Can you work these out from the model? Positions are in its coordinate system, mm. A direction names the side the tool comes from. Coordinates: 2 decimals unless noted, no trailing zeros. Order: outer loops, then holes, each group sorted by start corner. A loop starts at its lowest first (then second) coordinate and runs counter-clockwise, first axis right, second up. Notation, with made-up numbers: (49.5, 78) -> (84.5, 78) arc R35 ccw to (84.5, 114) -> close; hole circle Ø6 at (-18, 25). An arc over 180 degrees is marked (long way). Return JSON: item names as keys, results as strings. Group by question number.
1) If I drill on probe 1 along Y at (x, z) = (-17.5, 2.45); probe 2 along Y at (x, z) = (-12, 2.5); probe 3 along X at (y, z) = (27, 1.75), over which ranges is the centre line in solid material (lowest first)? Write a range as from..to.
2) If we section it at C-C, the plane z = 1.9: State how many separate pieces and enclosed holes the cut face has, then the cut area to 3 significant figures.
3) For pin 1 (1.5 mm diameter, centred on y = 46.5, z = 1.5, fed in from +X); pin 2 (1 mm diameter, centred on x = -18.5, z = 2, fed in from -Y); pin 3 (1 mm diameter, centred on y = -7.5, z = 1.5, fed in from -X), each with a flat end and sliding along its axis, tell me the tip position at first contact or that it passes through.
4) If we section it at A-A, the plane y = 19.2: Please give me the cut outline in (x, z) (3 decimals).
5) Thinking about a two-plate mould opening in X: for faces 3 (the cylindrical face through (-0.6, -8.93, 1.61)), 4 (the cylindrical face through (-19.66, 56.19, 2.1)), 5 (the cylindrical face through (-9.11, 6.47, 1.61)), which applies, +X half, -X half, draft (parallel to the pull), parting line (faces both ways), or undercut?
6) If we section it at D-D, the plane y = 4: Please give me the cut outline in (x, z) (3 decimals), then the cut area to 3 significant figures.
7) If we section it at B-B, the plane x = -12: Please give me the cut outline in (y, z) (3 decimals), then the cut area to 3 significant figures.
8) For faces 1 (the cylindrical face through (-19.41, 31.24, 2.1)), 2 (the flat face through (-20, 9.89, 2)), which set-ups out of +Z, -Z, +X, -X, +Y, -Y let a thin tool reach every point of the face, with its end or its side?
from build123d import *

# Parameters (mm, degrees)
SKETCH1_R                                       = 2.5
SKETCH1_R_2                                     = 5
SKETCH1_R_3                                     = 1
BOSS_EXTRUDE1_DEPTH                             = 3.175
CSK_FOR_M2_FLAT_HEAD_MACHINE_SCREW1_D           = 2.4
CSK_FOR_M2_FLAT_HEAD_MACHINE_SCREW1_CSINK_D     = 4.4
CSK_FOR_M2_FLAT_HEAD_MACHINE_SCREW1_CSINK_ANGLE = 90
SKETCH6_W                                       = 8
SKETCH6_H                                       = 3.2
MOTORSHAFTCUTOUT_DEPTH                          = 68.698453638
F_5MM_FILLET_R                                  = 5
F_1MM_FILLET_R                                  = 1
CUT_EXTRUDE1_DEPTH                              = 68.698453638
FILLET1_R                                       = 5
SKETCH8_W                                       = 5.5
SKETCH8_H                                       = 4
BOSS_EXTRUDE2_DEPTH                             = 3.175
BOSS_EXTRUDE3_DEPTH                             = 3.175
CUT_EXTRUDE3_DEPTH                              = 68.698453638
CUT_EXTRUDE3_DEPTH_BACK                         = 10
FILLET3_R                                       = 12
FILLET4_R                                       = 2
FILLET6_R                                       = 13
CSK_FOR_M2_FLAT_HEAD_MACHINE_SCREW3_D           = 2.4
CSK_FOR_M2_FLAT_HEAD_MACHINE_SCREW3_CSINK_D     = 4.4
CSK_FOR_M2_FLAT_HEAD_MACHINE_SCREW3_CSINK_ANGLE = 90


with BuildPart() as part:
    # Sketch1 → Boss-Extrude1 (new body)
    with BuildSketch(Plane.XY):
        with BuildLine():
            Line((0, -5.5), (-7, -5.5))
            Line((-7, -5.5), (-7, -9))
            Line((-7, -9), (-12, -9))
            Line((-12, -9), (-12, -2.5))
            Line((-12, -2.5), (-27, 4.494614872))
            Line((-27, 4.494614872), (-27, 62))
            Line((-27, 62), (-5, 62))
            Line((-5, 62), (-5, 32.19632141))
            Line((-5, 32.19632141), (-9, 28.19632141))
            Line((-9, 28.19632141), (-9, 10.265347478))
            Line((-9, 10.265347478), (2.32440044, 4.984692829))
            ThreePointArc((2.32440044, 4.984692829), (5.369628039, -1.190417877), (0, -5.5))
        make_face()
        Circle(SKETCH1_R, mode=Mode.SUBTRACT)
        with Locations((-18, 19.2)):
            Circle(SKETCH1_R_2, mode=Mode.SUBTRACT)
        with Locations((-16, 35.679077644)):
            Circle(SKETCH1_R_2, mode=Mode.SUBTRACT)
        with Locations((-9.5, 35.679077644)):
            Circle(SKETCH1_R_3, mode=Mode.SUBTRACT)
        with Locations((-19.25, 30.049912519)):
            Circle(SKETCH1_R_3, mode=Mode.SUBTRACT)
        with Locations((-19.25, 41.308242769)):
            Circle(SKETCH1_R_3, mode=Mode.SUBTRACT)
    extrude(amount=BOSS_EXTRUDE1_DEPTH)

    # CSK for M2 Flat Head Machine Screw1 (through all)
    with Locations(Plane(origin=(0, 0, 0), x_dir=(-1, 0, 0), z_dir=(0, 0, -1))):
        with Locations((19.5, 55), (12, 47.5)):
            CounterSinkHole(CSK_FOR_M2_FLAT_HEAD_MACHINE_SCREW1_D / 2, CSK_FOR_M2_FLAT_HEAD_MACHINE_SCREW1_CSINK_D / 2, counter_sink_angle=CSK_FOR_M2_FLAT_HEAD_MACHINE_SCREW1_CSINK_ANGLE)

    # Sketch6 → MotorShaftCutOut (cut, through all)
    with BuildSketch(Plane(origin=(0, 0, 0), x_dir=(-1, 0, 0), z_dir=(0, 0, -1))):
        with Locations((23, 35.7)):
            Rectangle(SKETCH6_W, SKETCH6_H)
    extrude(amount=-MOTORSHAFTCUTOUT_DEPTH, mode=Mode.SUBTRACT)

    # 5mm_Fillet
    f_5mm_fillet_edges = [part.edges().sort_by_distance(p)[0] for p in [
        (-12, -2.5, 1.5875),
        (-27, 4.494614872, 1.5875),
        (-27, 62, 1.5875),
        (-5, 62, 1.5875),
        (-5, 32.19632141, 1.5875),
        (-9, 28.19632141, 1.5875),
        (-9, 10.265347478, 1.5875),
    ]]
    fillet(f_5mm_fillet_edges, radius=F_5MM_FILLET_R)

    # 1mm_Fillet
    f_1mm_fillet_edges = [part.edges().sort_by_distance(p)[0] for p in [
        (-7, -5.5, 1.5875),
        (-7, -9, 1.5875),
        (-20.744103055, 34.1, 1.5875),
        (-20.72996942, 37.3, 1.5875),
        (-27, 34.1, 1.5875),
        (-27, 37.3, 1.5875),
    ]]
    fillet(f_1mm_fillet_edges, radius=F_1MM_FILLET_R)

    # Sketch7 → Cut-Extrude1 (cut, through all)
    with BuildSketch(Plane(origin=(0, 0, 0), x_dir=(-1, 0, 0), z_dir=(0, 0, -1))):
        with BuildLine():
            Line((12.047193362, -5), (17.277217948, 6.901547918))
            ThreePointArc((17.277217948, 6.901547918), (19.121399551, 9.076749311), (21.854736378, 9.89))
            Line((21.854736378, 9.89), (27, 9.89))
            Line((27, 9.89), (27, -5))
            Line((27, -5), (12.047193362, -5))
        make_face()
    extrude(amount=-CUT_EXTRUDE1_DEPTH, mode=Mode.SUBTRACT)

    # Fillet1
    fillet1_edges = [part.edges().sort_by_distance(p)[0] for p in [
        (-27, 9.89, 1.5875),
    ]]
    fillet(fillet1_edges, radius=FILLET1_R)

    # Sketch8 → Boss-Extrude2 (add)
    with BuildSketch(Plane(origin=(0, 0, 0), x_dir=(-1, 0, 0), z_dir=(0, 0, -1))):
        with Locations((2.75, -7.5)):
            Rectangle(SKETCH8_W, SKETCH8_H)
    extrude(amount=-BOSS_EXTRUDE2_DEPTH)

    # Sketch9 → Boss-Extrude3 (add)
    with BuildSketch(Plane.XY.offset(3.175)):
        with BuildLine():
            Line((-5, 34.267389222), (-5, 8.400116845))
            Line((-5, 8.400116845), (-6.113091309, 8.919159847))
            ThreePointArc((-6.113091309, 8.919159847), (-8.216957229, 10.76420074), (-9, 13.450698782))
            Line((-9, 13.450698782), (-9, 26.125253598))
            ThreePointArc((-9, 26.125253598), (-8.619397663, 28.03867076), (-7.535533906, 29.660787504))
            Line((-7.535533906, 29.660787504), (-6.464466094, 30.731855316))
            ThreePointArc((-6.464466094, 30.731855316), (-5.380602337, 32.35397206), (-5, 34.267389222))
        make_face()
    extrude(amount=-BOSS_EXTRUDE3_DEPTH)

    # Sketch10 → Cut-Extrude3 (cut, two sides: drawn at the far end of the back side and taken through both)
    with BuildSketch(Plane.XY.offset(3.175).offset(-CUT_EXTRUDE3_DEPTH_BACK)):
        with BuildLine():
            Line((-5.5, 9.89), (-21.854736378, 9.89))
            ThreePointArc((-21.854736378, 9.89), (-19.121399551, 9.076749311), (-17.277217948, 6.901547918))
            Line((-17.277217948, 6.901547918), (-13.145595024, -2.500455344))
            ThreePointArc((-13.145595024, -2.500455344), (-12.327289124, -3.906089359), (-12.003436692, -5.5))
            Line((-12.003436692, -5.5), (-6, -5.5))
            Line((-6, -5.5), (-5.5, -5.5))
            Line((-5.5, -5.5), (-5.5, 9.89))
        make_face()
    extrude(amount=CUT_EXTRUDE3_DEPTH + CUT_EXTRUDE3_DEPTH_BACK, mode=Mode.SUBTRACT)


with BuildPart() as body_2:
    # of the pieces the cut leaves, the one that is kept (cut_extrude3_keep)
    add(part.part.solids().sort_by_distance((-22, 9.89, 3.175))[0])

    # Fillet3
    fillet3_edges = [body_2.edges().sort_by_distance(p)[0] for p in [
        (-5.5, 9.89, 1.5875),
    ]]
    fillet(fillet3_edges, radius=FILLET3_R)

    # Fillet4
    fillet4_edges = [body_2.edges().sort_by_distance(p)[0] for p in [
        (0, -9.5, 1.5875),
    ]]
    fillet(fillet4_edges, radius=FILLET4_R)

    # Fillet6
    fillet6_edges = [body_2.edges().sort_by_distance(p)[0] for p in [
        (-5, 8.400116845, 1.5875),
    ]]
    fillet(fillet6_edges, radius=FILLET6_R)

    # CSK for M2 Flat Head Machine Screw3 (through all)
    with Locations(Plane(origin=(0, 0, 0), x_dir=(-1, 0, 0), z_dir=(0, 0, -1))):
        with Locations((19.25, 41.308242769), (9.5, 35.679077644), (19.25, 30.049912519)):
            CounterSinkHole(CSK_FOR_M2_FLAT_HEAD_MACHINE_SCREW3_D / 2, CSK_FOR_M2_FLAT_HEAD_MACHINE_SCREW3_CSINK_D / 2, counter_sink_angle=CSK_FOR_M2_FLAT_HEAD_MACHINE_SCREW3_CSINK_ANGLE)


solid = body_2.part
Result sheet:
{
 "1": {"probe 1": "y = 9.89..14.23, 24.17..30.91, 40.45..62", "probe 2": "y = 8.56..32.68, 38.68..46.3, 48.7..62", "probe 3": "x = -27..-5"},
 "2": {"separate pieces": "1", "enclosed holes": "7", "area": "1,090 mm2"},
 "3": {"pin 1": "stops at x = -5", "pin 2": "stops at y = 9.89", "pin 3": "stops at x = -5.5"},
 "4": {"outline": "(-27, 0) -> (-23, 0) -> (-23, 3.175) -> (-27, 3.175) -> close; (-13, 0) -> (-5, 0) -> (-5, 3.175) -> (-13, 3.175) -> close"},
 "5": {"face 3": "+X half", "face 4": "undercut", "face 5": "-X half"},
 "6": {"outline": "(-7.172, 0) -> (3.775, 0) -> (3.775, 3.175) -> (-7.172, 3.175) -> close", "area": "34.8 mm2"},
 "7": {"outline": "(8.555, 0) -> (32.679, 0) -> (32.679, 3.175) -> (8.555, 3.175) -> close; (38.679, 0) -> (45.3, 0) -> (46.3, 1) -> (46.3, 3.175) -> (38.679, 3.175) -> close; (48.7, 1) -> (49.7, 0) -> (62, 0) -> (62, 3.175) -> (48.7, 3.175) -> close", "area": "142 mm2"},
 "8": {"face 1": "+Z, -Z", "face 2": "+Z, -Z, -X, -Y"}
}
